The listing builds one solid part. Answer for the finished solid, in the listing's coordinates (mm). Give positions to 0.01 mm unless a question says otherwise; leave off trailing zeros. Order: outer loops, then holes, each group sorted by start corner. A loop starts at its lowest first (then second) coordinate and runs counter-clockwise, first axis right, second up. Notation, with made-up numbers: (54, 15) - (80, 15) arc R6 cw to (80, 23) - close; hole circle Ø4 at (4.25, -30.75). An arc over 180 degrees is marked (long way). Use CSV: the item, a comma, the result in double quotes.
```python
from build123d import *

# Parameters (mm, degrees)
EXTRUDE_1_DEPTH     = 2
SKETCH_3_W          = 10
SKETCH_3_H          = 54
EXTRUDE_2_DEPTH     = 2
SKETCH_2_R          = 1.55
CUT_EXTRUDE_1_DEPTH = 2
FILLET_1_R          = 3


with BuildPart() as part:
    # 草图1 → 凸台-拉伸1 (new body)
    with BuildSketch(Plane(origin=(0, 0, 0), x_dir=(1, 0, 0), z_dir=(0, 1, 0))):
        with BuildLine():
            Line((-59.5, -27), (-62.5, -27))
            Line((-62.5, -27), (-62.5, -24))
            Line((-62.5, -24), (-62.5, 24))
            Line((-62.5, 24), (-62.5, 27))
            Line((-62.5, 27), (-59.5, 27))
            Line((-59.5, 27), (59.5, 27))
            ThreePointArc((59.5, 27), (61.621320344, 26.121320344), (62.5, 24))
            Line((62.5, 24), (62.5, -24))
            ThreePointArc((62.5, -24), (61.621320344, -26.121320344), (59.5, -27))
            Line((59.5, -27), (-59.5, -27))
        make_face()
        with BuildLine():
            Line((-41.9, 21), (31.5, 21))
            ThreePointArc((31.5, 21), (32.207106781, 20.707106781), (32.5, 20))
            Line((32.5, 20), (32.5, -20))
            ThreePointArc((32.5, -20), (32.207106781, -20.707106781), (31.5, -21))
            Line((31.5, -21), (-41.9, -21))
            ThreePointArc((-41.9, -21), (-42.607106781, -20.707106781), (-42.9, -20))
            Line((-42.9, -20), (-42.9, 20))
            ThreePointArc((-42.9, 20), (-42.607106781, 20.707106781), (-41.9, 21))
        make_face(mode=Mode.SUBTRACT)
    extrude(amount=EXTRUDE_1_DEPTH)

    # 草图3 → 凸台-拉伸2 (add)
    with BuildSketch(Plane(origin=(0, 2, 0), x_dir=(1, 0, 0), z_dir=(0, 1, 0))):
        with Locations((-67.5, 0)):
            Rectangle(SKETCH_3_W, SKETCH_3_H)
    extrude(amount=-EXTRUDE_2_DEPTH)

    # 草图2 → 切除-拉伸1 (cut)
    with BuildSketch(Plane(origin=(0, 2, 0), x_dir=(1, 0, 0), z_dir=(0, 1, 0))):
        with Locations(Location((57.8, 23, 0), (0, 0, 270))):
            Circle(SKETCH_2_R)
        with Locations(Location((57.8, -23, 0), (0, 0, 90))):
            Circle(SKETCH_2_R)
        with Locations(Location((-67.8, -23, 0), (0, 0, 270))):
            Circle(SKETCH_2_R)
        with Locations(Location((-67.8, 23, 0), (0, 0, 90))):
            Circle(SKETCH_2_R)
    extrude(amount=-CUT_EXTRUDE_1_DEPTH, mode=Mode.SUBTRACT)

    # 圆角1
    fillet_1_edges = [part.edges().sort_by_distance(p)[0] for p in [
        (-72.5, 1, -27),
        (-72.5, 1, 27),
    ]]
    fillet(fillet_1_edges, radius=FILLET_1_R)


solid = part.part
```
Item 1: The mould has two halves that part along X. Classify faces 1 (the face through (-6, 0, 24)), 2 (the face through (56.263, 1.014, 23.202)), 3 (the face through (-71.64, 0.99, -26.1)): +X half, -X half, draft (parallel to the pull), parting line (faces both ways), or undercut.
Taken from the geometry:
face 1,"draft"
face 2,"undercut"
face 3,"-X half"
Item 2: The part is cut by section A-A (x = -7). Give the vertices of the cut face in (y, z).
Taken from the geometry:
outline,"(0, -27) - (2, -27) - (2, -21) - (0, -21) - close; (0, 21) - (2, 21) - (2, 27) - (0, 27) - close"
Item 3: The part is cut by section C-C (z = -18.5). Give the vertices of the cut face in (x, y).
Taken from the geometry:
outline,"(-72.5, 0) - (-42.9, 0) - (-42.9, 2) - (-72.5, 2) - close; (32.5, 0) - (62.5, 0) - (62.5, 2) - (32.5, 2) - close"
Item 4: Find the intervals of material crossed by line 1 along Z through (x, y) = (-67.8, 0.5); line 2 along X through (y, z) = (1.05, -23); line 3 along Z through (x, y) = (20.5, 0.6), in increasing order.
Taken from the geometry:
line 1,"-27 to -24.55, -21.45 to 21.45, 24.55 to 27"
line 2,"-72.5 to -69.35, -66.25 to 56.25, 59.35 to 62.5"
line 3,"-27 to -21, 21 to 27"
Item 5: The part is cut by section B-B (y = 1.7). Give the vertices of the cut face in (x, z).
Taken from the geometry:
outline,"(-72.5, -24) arc R3 ccw to (-69.5, -27) - (59.5, -27) arc R3 ccw to (62.5, -24) - (62.5, 24) arc R3 ccw to (59.5, 27) - (-69.5, 27) arc R3 ccw to (-72.5, 24) - close; hole circle Ø3.1 at (-67.8, -23); hole circle Ø3.1 at (-67.8, 23); hole (-42.9, -20) arc R1 ccw to (-41.9, -21) - (31.5, -21) arc R1 ccw to (32.5, -20) - (32.5, 20) arc R1 ccw to (31.5, 21) - (-41.9, 21) arc R1 ccw to (-42.9, 20) - close; hole circle Ø3.1 at (57.8, -23); hole circle Ø3.1 at (57.8, 23)"
Item 6: The part is cut by section D-D (x = 57.8). Give the vertices of the cut face in (y, z).
Taken from the geometry:
outline,"(0, -27) - (2, -27) - (2, -24.55) - (0, -24.55) - close; (0, -21.45) - (2, -21.45) - (2, 21.45) - (0, 21.45) - close; (0, 24.55) - (2, 24.55) - (2, 27) - (0, 27) - close"
Item 7: This flat-tipped pin is pushed along its axis until it touches: pin 1 (2.5 mm diameter, centred on x = 57.8, z = 23, fed in from +Y). Where does it stop, or does it pass through?
Taken from the geometry:
pin 1,"through"
